Autodesk Inventor part; units mm, degrees
ref_plane "YZ Plane" through (0, 0, 0) normal (1, 0, 0) x (0, 1, 0)
ref_plane "XZ Plane" through (0, 0, 0) normal (0, 1, 0) x (-1, 0, 0)
ref_plane "XY Plane" through (0, 0, 0) normal (0, 0, 1) x (1, 0, 0)
sketch "Sketch1" plane through (0, 0, 0) normal (0, 0, 1) x (1, 0, 0)
  line L0 (-63.5, -69.85) -> (63.5, -69.85)
  line L1 (69.85, -63.5) -> (69.85, 63.5)
  line L2 (63.5, 69.85) -> (-63.5, 69.85)
  line L3 (-69.85, 63.5) -> (-69.85, -63.5)
  arc A0 (-63.5, 69.85) -> (-69.85, 63.5) centre (-63.5, 63.5) ccw
  arc A1 (69.85, 63.5) -> (63.5, 69.85) centre (63.5, 63.5) ccw
  arc A2 (63.5, -69.85) -> (69.85, -63.5) centre (63.5, -63.5) ccw
  arc A3 (-69.85, -63.5) -> (-63.5, -69.85) centre (-63.5, -63.5) ccw
  point P0 (0, 0)
  point P1 (69.85, 0)
  point P2 (0, 69.85)
  point P3 (50.8, 50.8)
  dimension "d0" = 139.7
  dimension "d1" = 139.7
  dimension "d2" = 6.35
  dimension "d3" = 19.05
  dimension "d4" = 19.05
extrude "Extrusion1" add sketch "Sketch1" against normal blind 6.35
hole "Hole1" at (-63.5, 63.5, 0) at (63.5, 63.5, 0) at (63.5, -63.5, 0) at (-63.5, -63.5, 0) direction (0, 0, -1) diameter 4.4958 end through all
hole "Hole2" at (50.8, 50.8, 0) direction (0, 0, -1) diameter 3.9624 end through all
equation "\"d1\" = d0"
properties part number "J007954" material "ACRYLIC, CLEAR"
CAD build for the part. Positions are in the model's coordinates, mm. Give positions to 0.01 mm unless a question says otherwise; leave off trailing zeros. Loops run counter-clockwise (first coordinate to the right, second up) from the corner with the lowest first, then second, coordinate; pieces in that order, holes last. Notation, with made-up numbers: M 86.5,-12 L 110.5,-12 A19 ccw 110.5,7 Z; hole C -34.5,18 d3. An arc over 180 degrees is marked long. Answer in a Markdown table with one row per item. Add a question column.
Item 1: Probe probe 1 along X at (y, z) = (63.5, -4.25); probe 2 along Y at (x, z) = (50.8, -2.5). List the from-to ranges inside material, lowest first.
Item 2: Mould opens along Y. For faces 1 (the face through (-62.13, -61.72, -3.22)), 2 (the face through (-1, -69.85, -3)), 3 (the face through (-69.85, 1, -3)) say: +Y half, -Y half, draft (parallel to the pull), parting line (faces both ways), or undercut.
Item 3: Band-saw the part on A-A on y = 50.8. Give the cut face in (x, z), then the cut area to 3 significant figures.
Reply:
| question | item | result |
|---|---|---|
| 1 | probe 1 | x = -69.85 to -65.75, -61.25 to 61.25, 65.75 to 69.85 |
| 1 | probe 2 | y = -69.85 to 48.82, 52.78 to 69.85 |
| 2 | face 1 | undercut |
| 2 | face 2 | -Y half |
| 2 | face 3 | draft |
| 3 | outline | M -69.85,-6.35 L 48.82,-6.35 L 48.82,0 L -69.85,0 Z; M 52.78,-6.35 L 69.85,-6.35 L 69.85,0 L 52.78,0 Z |
| 3 | area | 862 mm^2 |
